Read the model definition and answer for the solid it produces. Units are mm, in the model's axes. A direction names the side the tool comes from. Give positions to 0.01 mm unless a question says otherwise; leave off trailing zeros. Loops run counter-clockwise (first coordinate to the right, second up) from the corner with the lowest first, then second, coordinate; pieces in that order, holes last. Notation, with made-up numbers: (-6.5, -30.75) -> (43.5, -30.75) arc R4 cw to (43.5, -26.75) -> close; hole circle Ø6 at (-16, 43.25). An arc over 180 degrees is marked (long way). Answer as CSV lines item,"result". Start each with the question number.
```python
from build123d import *

# Parameters (mm, degrees)
BOSS_EXTRUDE1_OUTLINE_W   = 30
BOSS_EXTRUDE1_OUTLINE_H   = 20
BOSS_EXTRUDE1_OUTLINE_W_2 = 25
BOSS_EXTRUDE1_OUTLINE_H_2 = 15
BOSS_EXTRUDE1_DEPTH       = 20
SKETCH4_R                 = 1.5
CUT_EXTRUDE3_DEPTH        = 38.416573868
FILLET1_R                 = 5


# Read off the part's stored shape, not the designer's step: Boss-Extrude1
with BuildPart() as part:
    # Boss-Extrude1 outline → Boss-Extrude1 (new body)
    with BuildSketch(Plane(origin=(0, 0, 0), x_dir=(1, 0, 0), z_dir=(0, 1, 0))):
        Rectangle(BOSS_EXTRUDE1_OUTLINE_W, BOSS_EXTRUDE1_OUTLINE_H)
        Rectangle(BOSS_EXTRUDE1_OUTLINE_W_2, BOSS_EXTRUDE1_OUTLINE_H_2, mode=Mode.SUBTRACT)
    extrude(amount=BOSS_EXTRUDE1_DEPTH)

    # Sketch4 → Cut-Extrude3 (cut, through all)
    with BuildSketch(Plane(origin=(15, 0, 0), x_dir=(0, 0, -1), z_dir=(1, 0, 0))):
        with Locations((0, 16)):
            Circle(SKETCH4_R)
        with Locations((0, 4)):
            Circle(SKETCH4_R)
    extrude(amount=-CUT_EXTRUDE3_DEPTH, mode=Mode.SUBTRACT)

    # Fillet1
    fillet1_edges = [part.edges().sort_by_distance(p)[0] for p in [
        (12.5, 10, 7.5),
        (12.5, 10, -7.5),
        (-12.5, 10, -7.5),
        (-12.5, 10, 7.5),
    ]]
    fillet(fillet1_edges, radius=FILLET1_R)


solid = part.part
```
(1) Find section B-B on y = 1.5. Write down the section's boundary in (x, z).
(2) Find section A-A on z = -5.5. Write down the section's boundary in (x, y), then the cut area to 3 significant figures.
(3) A tool of negligible diameter and unlimited length cuts with its end or side. For faces 4 (the face through (0, 10, 10)), 5 (the face through (0, 10, -7.5)), from which of +Z, -Z, +X, -X, +Y, -Y can it reach the whole face along a straight path? Write none if from no direction.
(4) Find section D-D on z = 0. Write down the section's boundary in (x, y), then the cut area to 3 significant figures.
(5) Find section C-C on x = -4.25. Write down the section's boundary in (y, z).
(6) Find the intervals of material crossed by line 1 along Y through (x, z) = (14, 0); line 2 along X through (y, z) = (10.75, -1); line 3 along Z through (x, y) = (4, 6), in increasing order. Write a range as from..to.
(7) This flat-tipped pin is pushed along its axis until it touches: P1, Ø1, axis at x = 7.5, z = 5, coming from the -Y side. Where does it stop, or does it pass through?
(8) The mould has two halves that part along Z. Classify faces 1 (the face through (0, 0, -9)), 2 (the face through (0, 10, -10)), 3 (the face through (11, 10.14, 6.07)): pulls with the +Z half, pulls with the -Z half, needs draft (parallel to the pull), parting line crosses it, or undercut.
Answer block:
1,outline,"(-15, -10) -> (15, -10) -> (15, 10) -> (-15, 10) -> close; hole (-12.5, -2.5) arc R5 ccw to (-7.5, -7.5) -> (7.5, -7.5) arc R5 ccw to (12.5, -2.5) -> (12.5, 2.5) arc R5 ccw to (7.5, 7.5) -> (-7.5, 7.5) arc R5 ccw to (-12.5, 2.5) -> close"
2,outline,"(-15, 0) -> (-11.5, 0) -> (-11.5, 20) -> (-15, 20) -> close; (11.5, 0) -> (15, 0) -> (15, 20) -> (11.5, 20) -> close"
2,area,"140 mm2"
3,face 4,"+Z, +X, -X, +Y, -Y"
3,face 5,"+Y, -Y"
4,outline,"(-15, 0) -> (-12.5, 0) -> (-12.5, 2.5) -> (-15, 2.5) -> close; (-15, 5.5) -> (-12.5, 5.5) -> (-12.5, 14.5) -> (-15, 14.5) -> close; (-15, 17.5) -> (-12.5, 17.5) -> (-12.5, 20) -> (-15, 20) -> close; (12.5, 0) -> (15, 0) -> (15, 2.5) -> (12.5, 2.5) -> close; (12.5, 5.5) -> (15, 5.5) -> (15, 14.5) -> (12.5, 14.5) -> close; (12.5, 17.5) -> (15, 17.5) -> (15, 20) -> (12.5, 20) -> close"
4,area,"70.0 mm2"
5,outline,"(0, -10) -> (20, -10) -> (20, -7.5) -> (0, -7.5) -> close; (0, 7.5) -> (20, 7.5) -> (20, 10) -> (0, 10) -> close"
6,line 1,"y = 0..2.5, 5.5..14.5, 17.5..20"
6,line 2,"x = -15..-12.5, 12.5..15"
6,line 3,"z = -10..-7.5, 7.5..10"
7,P1,"passes through"
8,face 1,"needs draft"
8,face 2,"pulls with the -Z half"
8,face 3,"undercut"
